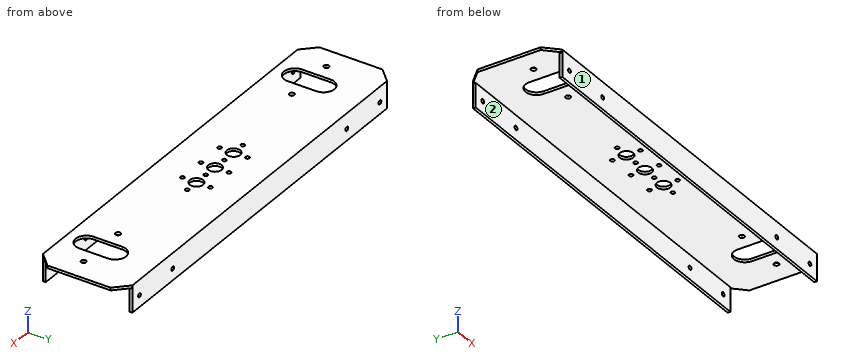
Autodesk Inventor part; units mm, degrees
ref_plane "YZ Plane" through (0, 0, 0) normal (1, 0, 0) x (0, 1, 0)
ref_plane "XZ Plane" through (0, 0, 0) normal (0, 1, 0) x (-1, 0, 0)
ref_plane "XY Plane" through (0, 0, 0) normal (0, 0, 1) x (1, 0, 0)
sketch "Sketch1" plane through (0, 0, 0) normal (0, 0, 1) x (1, 0, 0)
  line L0 (-114.2436, 26.55) -> (114.2436, 26.55)
  line L1 (122, 18.7501) -> (122, -18.7501)
  line L2 (114.2436, -26.55) -> (-114.2436, -26.55)
  line L3 (-122, -18.7501) -> (-122, 18.7501)
  line L4 (114.2436, 26.55) -> (122, 18.7501)
  line L5 (122, -18.7501) -> (114.2436, -26.55)
  line L6 (0, 26.55) -> (0, -26.55)
  line L7 (-114.2436, 26.55) -> (-122, 18.7501)
  line L8 (-122, -18.7501) -> (-114.2436, -26.55)
  point P0 (0, 0)
  point P1 (-122, 0)
  point P2 (0, 26.55)
  point P3 (0, 0)
  dimension "d0" = 244
  dimension "d62" = 135.16
  dimension "d63" = 11
  dimension "d64" = 135.16
  dimension "d65" = 11
  dimension "d66" = 53.1
extrude "Extrusion5" add sketch "Sketch1" along normal blind 1.6
sketch "Sketch11" plane through (-114.2436, 26.55, 0) normal (0, 1, 0) x (1, 0, 0)
  line L0 (228.4872, 0) -> (0, 0)
  line L1 (0, 0) -> (0, -1.6)
  line L2 (228.4872, -1.6) -> (0, -1.6)
  line L3 (228.4872, 0) -> (228.4872, -1.6)
  line L4 (228.4872, 0) -> (0, 0)
  line L5 (0, 0) -> (228.4872, 0)
  line L6 (228.4872, 0) -> (228.4872, 14.4)
  line L7 (228.4872, 14.4) -> (0, 14.4)
  line L8 (0, 14.4) -> (0, 0)
  point P0 (114.2436, 0)
  dimension "d72" = 14.4
extrude "Extrusion6" add sketch "Sketch11" against normal blind 1.6 contours L0 L8 L7 L6
sketch "Sketch12" plane through (-114.2436, -26.55, 0) normal (0, -1, 0) x (1, 0, 0)
  line L0 (228.4872, -14.4) -> (228.4872, 0)
  line L1 (0, 0) -> (228.4872, 0)
  line L2 (0, 0) -> (0, -14.4)
  line L3 (0, -14.4) -> (228.4872, -14.4)
  line L4 (0, 0) -> (228.4872, 0)
  line L5 (0, 0) -> (228.4872, 0)
  line L6 (228.4872, 0) -> (228.4872, -14.4)
  line L7 (228.4872, -14.4) -> (0, -14.4)
  line L8 (0, -14.4) -> (0, 0)
  point P0 (114.2436, 0)
extrude "Extrusion7" add sketch "Sketch12" against normal blind 1.6
sketch "Sketch13" plane through (-114.2436, 26.55, 1.6) normal (0, 1, 0) x (1, 0, 0)
  line L0 (0, 1.6) -> (0, 0)
  line L1 (228.4872, 0) -> (0, 0)
  line L2 (228.4872, 1.6) -> (228.4872, 0)
  line L3 (228.4872, 1.6) -> (228.4872, 16)
  line L4 (228.4872, 16) -> (0, 16)
  line L5 (0, 16) -> (0, 1.6)
  line L6 (228.4872, 16) -> (0, 16) construction
  line L7 (114.2436, 16) -> (114.2436, 0) construction
  line L8 (36.1513, 9.1) -> (114.2436, 9.1) construction
  line L9 (114.2436, 9.1) -> (192.3359, 9.1) construction
  point P0 (114.2436, 1.6)
  point P1 (0, 8.8)
  point P2 (6.354, 9.1)
  point P3 (222.1332, 9.1)
  dimension "d79" = 6.354
  dimension "d80" = 6.354
  dimension "d110" = 6.9
  dimension "d111" = 6.9
  dimension "d112" = 156.1846
hole "Hole6" at (-78.0923, 26.55, -7.5) at (78.0923, 26.55, -7.5) at (-107.8896, 26.55, -7.5) at (107.8896, 26.55, -7.5) direction (0, -1, 0) diameter 2.459 end up to surface
sketch "Sketch14" plane through (-114.2436, -26.55, 1.6) normal (0, -1, 0) x (1, 0, 0)
  circle A0 centre (192.3359, -9.1) radius 1.2295
  circle A1 centre (222.1332, -9.1) radius 1.2295
  circle A2 centre (36.1513, -9.1) radius 1.2295
  circle A3 centre (6.354, -9.1) radius 1.2295
  point P0 (114.2436, -1.6)
hole "Hole7" at (-107.8896, -26.55, -7.5) at (-78.0923, -26.55, -7.5) at (78.0923, -26.55, -7.5) at (107.8896, -26.55, -7.5) direction (0, 1, 0) diameter 2.459 end up to surface
sketch "Sketch15" plane through (0, 0, 1.6) normal (0, 0, 1) x (1, 0, 0)
  line L0 (-93.5, 2.55) -> (-93.5, -14.45) construction
  line L1 (-100, 2.55) -> (-100, -14.45)
  line L2 (-87, -14.45) -> (-87, 2.55)
  arc A0 (-87, 2.55) -> (-100, 2.55) centre (-93.5, 2.55) ccw
  arc A1 (-100, -14.45) -> (-87, -14.45) centre (-93.5, -14.45) ccw
  line L3 (-122, 18.7501) -> (-122, -18.7501)
  line L4 (114.2436, 26.55) -> (-114.2436, 26.55)
  line L5 (0, 26.55) -> (0, -26.55)
  line L6 (-114.2436, -26.55) -> (114.2436, -26.55)
  line L7 (93.5, 2.55) -> (93.5, -14.45) construction
  line L8 (100, 2.55) -> (100, -14.45)
  line L9 (87, -14.45) -> (87, 2.55)
  arc A2 (100, 2.55) -> (87, 2.55) centre (93.5, 2.55) ccw
  arc A3 (87, -14.45) -> (100, -14.45) centre (93.5, -14.45) ccw
  point P0 (0, 0)
  point P1 (-93.5, -5.95)
  point P2 (93.5, -5.95)
  dimension "d95" = 17
  dimension "d96" = 13
  dimension "d97" = 22
  dimension "d98" = 24
extrude "Extrusion8" cut sketch "Sketch15" against normal through all
sketch "Sketch16" plane through (0, 0, 1.6) normal (0, 0, 1) x (1, 0, 0)
  line L0 (-109, -5.95) -> (-78, -5.95)
  line L1 (78, -5.95) -> (109, -5.95)
  arc A0 (-87, 2.55) -> (-100, 2.55) centre (-93.5, 2.55) ccw
  arc A1 (100, 2.55) -> (87, 2.55) centre (93.5, 2.55) ccw
  line L2 (-87, 2.55) -> (-87, -14.45)
  point P0 (0, 0)
  point P1 (-93.5, -5.95)
  point P2 (93.5, -5.95)
  point P3 (-87, -5.95)
  dimension "d101" = 31
  dimension "d102" = 31
hole "Hole8" at (-109, -5.95, 1.6) at (-78, -5.95, 1.6) at (78, -5.95, 1.6) at (109, -5.95, 1.6) direction (0, 0, -1) diameter 3 end through all
sketch "Sketch17" plane through (0, 0, 1.6) normal (0, 0, 1) x (1, 0, 0)
  circle A0 centre (0, 0) radius 4.0005
  circle A1 centre (0, 8.3312) radius 1.1938
  circle A2 centre (-8.3312, 0) radius 1.1938
  circle A3 centre (0, -8.3312) radius 1.1938
  circle A4 centre (8.3312, 0) radius 1.1938
  circle A5 centre (-16.6624, 0) radius 4.0005
  circle A6 centre (-16.6624, 8.3312) radius 1.1938
  circle A7 centre (-24.9936, 0) radius 1.1938
  circle A8 centre (-16.6624, -8.3312) radius 1.1938
  circle A9 centre (-8.3312, 0) radius 1.1938
  circle A10 centre (16.6624, 0) radius 4.0005
  circle A11 centre (16.6624, 8.3312) radius 1.1938
  circle A12 centre (8.3312, 0) radius 1.1938
  circle A13 centre (16.6624, -8.3312) radius 1.1938
  circle A14 centre (24.9936, 0) radius 1.1938
  circle A15 centre (78, -5.95) radius 1.5
  circle A16 centre (-109, -5.95) radius 1.5
  circle A17 centre (-78, -5.95) radius 1.5
  circle A18 centre (109, -5.95) radius 1.5
  arc A19 (-100, -14.45) -> (-87, -14.45) centre (-93.5, -14.45) ccw
  line L0 (-100, -14.45) -> (-100, 2.55)
  arc A20 (-87, 2.55) -> (-100, 2.55) centre (-93.5, 2.55) ccw
  line L1 (-87, 2.55) -> (-87, -14.45)
  arc A21 (87, -14.45) -> (100, -14.45) centre (93.5, -14.45) ccw
  line L2 (87, -14.45) -> (87, 2.55)
  arc A22 (100, 2.55) -> (87, 2.55) centre (93.5, 2.55) ccw
  line L3 (100, 2.55) -> (100, -14.45)
  line L4 (122, -18.7501) -> (122, 18.7501)
  line L5 (122, 18.7501) -> (114.2436, 26.55)
  line L6 (114.2436, 26.55) -> (-114.2436, 26.55)
  line L7 (-114.2436, 26.55) -> (-122, 18.7501)
  line L8 (-122, 18.7501) -> (-122, -18.7501)
  line L9 (-122, -18.7501) -> (-114.2436, -26.55)
  line L10 (-114.2436, -26.55) -> (114.2436, -26.55)
  line L11 (114.2436, -26.55) -> (122, -18.7501)
  point P0 (0, 18.8)
  point P1 (0, 37.6)
  point P2 (201.549, 0)
  point P3 (0, 18.8)
  point P4 (0, 26.55)
  point P5 (-122, 0)
  dimension "d113" = 8.001
  dimension "d114" = 8.3312
  dimension "d115" = 2.3876
  dimension "d116" = 360
  dimension "d117" = 8.001
  dimension "d118" = 8.3312
  dimension "d119" = 2.3876
  dimension "d120" = 360
  dimension "d121" = 8.001
  dimension "d122" = 8.3312
  dimension "d123" = 2.3876
  dimension "d124" = 360
  dimension "d125" = 16.6624
  dimension "d126" = 16.6624
  dimension "d130" = 43.1852
  dimension "d131" = 82.0064
  dimension "d132" = 73.216
  dimension "d133" = 86.4724
extrude "Extrusion9" cut sketch "Sketch17" against normal through all contours A0 | A1 | A2 | A3 | A4 | A5 | A6 | A7 | A8 | A10 | A11 | A13 | A14
equation "\"d64\" = d62"
equation "\"d111\" = d110"
equation "\"d126\" = d125"
properties part number "ChassisSideBracket"
Geometry: final body of the model. Coordinates: model frame, mm. Face numbers are marked on the shaded views. A direction names the side the tool comes from. Round coordinates to 2 decimals unless told otherwise and drop trailing zeros. Loops run counter-clockwise (first coordinate to the right, second up) from the corner with the lowest first, then second, coordinate; pieces in that order, holes last. Notation, with made-up numbers: M 59,-12 L 65,-12 A21 cw 65,13 Z; hole C 86.25,21 d9. An arc over 180 degrees is marked long. One line per question, with ' | ' between items.
(1) Material intervals for line 1 along Y through (x, z) = (-86, -12.5); line 2 along X through (y, z) = (25.45, -7.5); line 3 along Z through (x, y) = (66, 0.5), sorted ascending. Write a range as from..to.
Check result:
line 1: y = -26.55..-24.95, 24.95..26.55 | line 2: x = -114.24..-109.12, -106.66..-79.32, -76.86..76.86, 79.32..106.66, 109.12..114.24 | line 3: z = 0..1.6
(2) Cut plane B-B on x = 29. Return the cut outline in (y, z).
Check result:
outline: M -26.55,-14.4 L -24.95,-14.4 L -24.95,0 L 24.95,0 L 24.95,-14.4 L 26.55,-14.4 L 26.55,1.6 L -26.55,1.6 Z
(3) Access query for the marked faces 1 and 2. Directions: +Z, -Z, +X, -X, +Y, -Y. A direction counts if a zero-diameter tool reaches every point of the face in a straight line with its end or side. Return the directions, or none.
Check result:
face 1: +Z, -Z, +X, -X, -Y | face 2: -Z, +X, -X
(4) Cut plane A-A on z = -11.5. Return the cut outline in (x, y).
Check result:
outline: M -114.24,-26.55 L 114.24,-26.55 L 114.24,-24.95 L -114.24,-24.95 Z; M -114.24,24.95 L 114.24,24.95 L 114.24,26.55 L -114.24,26.55 Z
(5) Contact query for flat-ended pins moving along their axis: P1, Ø2.5, axis at x = 16.66, y = 8.33, coming from the -Z side; P2, Ø2, axis at x = -8.33, y = 0, coming from the -Z side; P3, Ø0.5, axis at y = 26, z = -10, coming from the -X side. Output: stop coordinate, or through.
Check result:
P1: stops at z = 0 | P2: passes through | P3: stops at x = -114.24
(6) Cut plane C-C on y = 15. Return the cut outline in (x, z), plus the area to 3 significant figures.
Check result:
outline: M -122,0 L 122,0 L 122,1.6 L -122,1.6 Z | area: 390 mm2
